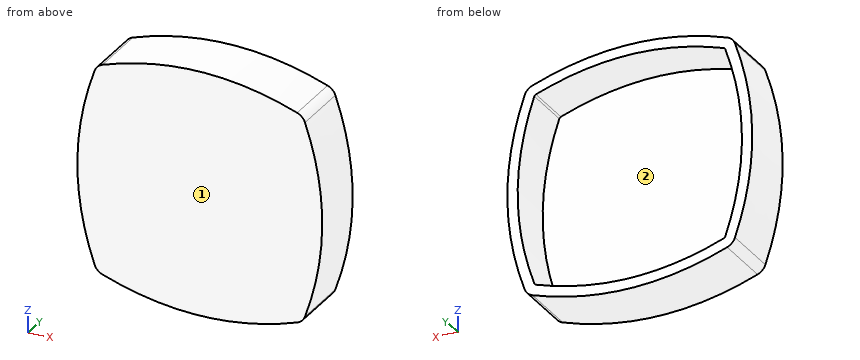
from build123d import *

# Parameters (mm, degrees)
BOSS_EXTRUDE1_DEPTH = 14.2875
FILLET1_R           = 3.175
SHELL1_T            = -2.54


with BuildPart() as part:
    # Sketch1 → Boss-Extrude1 (new body)
    with BuildSketch(Plane(origin=(0, 0, 0), x_dir=(1, 0, 0), z_dir=(0, 1, 0))):
        with BuildLine():
            Line((0, 0), (-30.1625, 0))
            add(Edge.make_bspline(
                [(-30.1625, 0), (-30.1625, -12.7), (-25.4, -25.4)],
                knots=[0.5, 0.5, 0.5, 1, 1, 1], degree=2))
            add(Edge.make_bspline(
                [(-25.4, -25.4), (-12.7, -30.1625), (0, -30.1625)],
                knots=[0, 0, 0, 0.5, 0.5, 0.5], degree=2))
            Line((0, -30.1625), (0, 0))
        make_face()
        with BuildLine():
            add(Edge.make_bspline(
                [(-25.4, 25.4), (-30.1625, 12.7), (-30.1625, 0)],
                knots=[0, 0, 0, 0.5, 0.5, 0.5], degree=2))
            Line((-30.1625, 0), (0, 0))
            Line((0, 0), (0, 30.1625))
            add(Edge.make_bspline(
                [(-25.4, 25.4), (-12.7, 30.1625), (0, 30.1625)],
                knots=[0, 0, 0, 0.5, 0.5, 0.5], degree=2))
        make_face()
        with BuildLine():
            Line((0, 30.1625), (0, 0))
            Line((0, 0), (30.1625, 0))
            add(Edge.make_bspline(
                [(25.4, 25.4), (30.1625, 12.7), (30.1625, 0)],
                knots=[0, 0, 0, 0.5, 0.5, 0.5], degree=2))
            add(Edge.make_bspline(
                [(0, 30.1625), (12.7, 30.1625), (25.4, 25.4)],
                knots=[0.5, 0.5, 0.5, 1, 1, 1], degree=2))
        make_face()
        with BuildLine():
            Line((30.1625, 0), (0, 0))
            Line((0, 0), (0, -30.1625))
            add(Edge.make_bspline(
                [(0, -30.1625), (12.7, -30.1625), (25.4, -25.4)],
                knots=[0.5, 0.5, 0.5, 1, 1, 1], degree=2))
            add(Edge.make_bspline(
                [(30.1625, 0), (30.1625, -12.7), (25.4, -25.4)],
                knots=[0.5, 0.5, 0.5, 1, 1, 1], degree=2))
        make_face()
    extrude(amount=BOSS_EXTRUDE1_DEPTH)

    # Fillet1
    fillet1_edges = [part.edges().sort_by_distance(p)[0] for p in [
        (-25.4, 7.14375, -25.4),
        (25.4, 7.14375, -25.4),
        (-25.4, 7.14375, 25.4),
        (25.4, 7.14375, 25.4),
    ]]
    fillet(fillet1_edges, radius=FILLET1_R)

    # Shell1
    shell1_openings = [part.faces().sort_by_distance(p)[0] for p in [
        (0, 14.2875, 0),
    ]]
    offset(amount=SHELL1_T, openings=shell1_openings, kind=Kind.INTERSECTION)


solid = part.part
Can you work these out from the model? Positions are in its coordinate system, mm. Face numbers are marked on the shaded views. Round coordinates to 2 decimals unless told otherwise and drop trailing zeros. Use a Markdown table: item, result.
1) If I drill on line 1 along Y through (x, z) = (-21.5, -15); line 2 along Z through (x, y) = (-19, 5); line 3 along X through (y, z) = (11.5, 6), over which ranges is the centre line in solid material (lowest first)?
Geometry says:
| item | result |
|---|---|
| line 1 | y = 0 to 2.54 |
| line 2 | z = -27.5 to -24.86, 24.86 to 27.5 |
| line 3 | x = -29.9 to -27.35, 27.35 to 29.9 |
2) If we mould it in two halves opening along Z, with no side actions, what happens to the marked faces 1 and 2? For each: +Z half, -Z half, draft (parallel to the pull), parting line (faces both ways), or undercut.
Geometry says:
| item | result |
|---|---|
| face 1 | draft |
| face 2 | undercut |
3) I'm going to push flat-ended pins straight in: P1, Ø6, axis at y = 11, z = 17.5, coming from the +X side; P2, Ø8, axis at x = -9, y = 3, coming from the -Z side; P3, Ø10, axis at x = 17, z = -15, coming from the -Y side; P4, Ø1.5, axis at y = 8, z = -13.5, coming from the -X side. Where does each tip first touch, or does it pass through?
Geometry says:
| item | result |
|---|---|
| P1 | stops at x = 28.61 |
| P2 | stops at z = -29.98 |
| P3 | stops at y = 0 |
| P4 | stops at x = -28.96 |
